```python
from build123d import *

# Parameters (mm, degrees)
BOSS_EXTRUDE2_DEPTH = 2
SKETCH3_R           = 1.5
CUT_EXTRUDE2_DEPTH  = 5


with BuildPart() as part:
    # Sketch1 → Revolve1 (revolve)
    with BuildSketch(Plane.XY, mode=Mode.PRIVATE) as revolve1_sk:
        Polygon((0, 0), (-5, 0), (-5, 3), (-1.5, 3), (-1.5, 6), (-5, 6), (-5, 7.1), (-1, 7.1), (-1, 6), (1, 6), (1, 7.1), (5, 7.1), (5, 6), (1.5, 6), (1.5, 0), align=None)
    revolve(revolve1_sk.sketch.rotate(Axis((1.5, 0, 0), (-1, 0, 0)), 90), axis=Axis((1.5, 0, 0), (-1, 0, 0)))

    # Sketch2 → Boss-Extrude2 (add)
    with BuildSketch(Plane(origin=(0, 0, 0), x_dir=(0, 0, -1), z_dir=(1, 0, 0))):
        with BuildLine():
            Line((0.5, 1.936491673), (0.5, 5.979130372))
            ThreePointArc((0.5, 5.979130372), (0, 6), (-0.5, 5.979130372))
            Line((-0.5, 5.979130372), (-0.5, 1.936491673))
            ThreePointArc((-0.5, 1.936491673), (-1.414213562, 1.414213562), (-1.936491673, 0.5))
            Line((-1.936491673, 0.5), (-5.979130372, 0.5))
            ThreePointArc((-5.979130372, 0.5), (-6, 0), (-5.979130372, -0.5))
            Line((-5.979130372, -0.5), (-1.936491673, -0.5))
            ThreePointArc((-1.936491673, -0.5), (-1.414213562, -1.414213562), (-0.5, -1.936491673))
            Line((-0.5, -1.936491673), (-0.5, -5.979130372))
            ThreePointArc((-0.5, -5.979130372), (0, -6), (0.5, -5.979130372))
            Line((0.5, -5.979130372), (0.5, -1.936491673))
            ThreePointArc((0.5, -1.936491673), (1.414213562, -1.414213562), (1.936491673, -0.5))
            Line((1.936491673, -0.5), (5.979130372, -0.5))
            ThreePointArc((5.979130372, -0.5), (6, 0), (5.979130372, 0.5))
            Line((5.979130372, 0.5), (1.936491673, 0.5))
            ThreePointArc((1.936491673, 0.5), (1.414213562, 1.414213562), (0.5, 1.936491673))
        make_face()
    extrude(amount=BOSS_EXTRUDE2_DEPTH)

    # Sketch3 → Cut-Extrude2 (cut)
    with BuildSketch(Plane.ZY.offset(5)):
        Circle(SKETCH3_R)
    extrude(amount=-CUT_EXTRUDE2_DEPTH, mode=Mode.SUBTRACT)


solid = part.part
```
Read the model definition and answer for the solid it produces. Units are mm, in the model's axes. A direction names the side the tool comes from. Round coordinates to 2 decimals unless told otherwise and drop trailing zeros. Write each loop counter-clockwise with the first axis right and the second up, starting at its lowest first coordinate (ties: lowest second). Pieces come first, ordered by that corner, then holes. Notation, with made-up numbers: (74, -39.75) - (107, -39.75) arc R20 cw to (107, -33.75) - close; hole circle Ø3 at (-5, -23.75). An arc over 180 degrees is marked (long way). One line per item, written item: value.
Q1. Which of the six approach directions +Z, -Z, +X, -X, +Y, -Y give full straight-line access (tool end or side, diameter ignored) to faces 4 (the flat face through (1, -6, -2)), 5 (the cylindrical face through (1.746, -1.404, 1.425)), 6 (the flat face through (-5, 1.3, 1.3)), 7 (the flat face through (0, 0, 0))?
The answers:
face 4: none
face 5: +X
face 6: +Z, -Z, -X, +Y, -Y
face 7: -X
Q2. Straight lines are drawn through the part: line 1 (Y direction, x = -3.5, z = 0); line 2 (Y direction, x = 1.75, z = 4.75); line 3 (Z direction, x = -3.5, y = 0.25). For each, find the intervals that lie inside material, in ascending order. Write a range as from..to.
The answers:
line 1: y = -7.1..-6, -3..-1.5, 1.5..3, 6..7.1
line 2: y = -5.28..-3.67, -0.5..0.5, 3.67..5.28
line 3: z = -7.1..-5.99, -2.99..-1.48, 1.48..2.99, 5.99..7.1
Q3. Find section A-A (y = 0). Determine the outline of the cut face in (x, z).
The answers:
outline: (-5, -7.1) - (-1, -7.1) - (-1, -6) - (1, -6) - (1, -7.1) - (5, -7.1) - (5, -6) - (2, -6) - (2, 6) - (5, 6) - (5, 7.1) - (1, 7.1) - (1, 6) - (-1, 6) - (-1, 7.1) - (-5, 7.1) - (-5, 6) - (-1.5, 6) - (-1.5, 3) - (-5, 3) - (-5, 1.5) - (0, 1.5) - (0, -1.5) - (-5, -1.5) - (-5, -3) - (-1.5, -3) - (-1.5, -6) - (-5, -6) - close
Q4. Find section B-B (x = -2.5). Determine the outline of the cut face in (y, z), and give its area (3 significant figures).
The answers:
outline: circle Ø14.2 at (0, 0); circle Ø6 at (0, 0); hole circle Ø12 at (0, 0); hole circle Ø3 at (0, 0)
area: 66.5 mm2
Q5. Find section D-D (x = 4). Determine the outline of the cut face in (y, z), and give its area (3 significant figures).
The answers:
outline: circle Ø14.2 at (0, 0); hole circle Ø12 at (0, 0)
area: 45.3 mm2
Q6. Each of these flat-tipped pins is pushed along its axis until it touches: P1, Ø2.5, axis at y = 3, z = -2, coming from the +X side; P2, Ø3, axis at x = 3.5, z = -1, coming from the -Y side; P3, Ø6, axis at y = -0.5, z = -0.5, coming from the +X side; P4, Ø3, axis at x = 4, z = -5.5, coming from the -Y side. Where does it stop, or does it pass through?
The answers:
P1: stops at x = 1.5
P2: stops at y = -7.1
P3: stops at x = 2
P4: stops at y = -5.87
Q7. For a pull along Y with two mould halves and no side action, classify faces 1 (the flat face through (1.5, -3, -3)), 2 (the cylindrical face through (-2.97, -7.04, 0.92)), 3 (the flat face through (5, -6, 2)) as pulls with the +Y half, pulls with the -Y half, needs draft (parallel to the pull), parting line crosses it, or undercut.
The answers:
face 1: undercut
face 2: parting line crosses it
face 3: needs draft
